from build123d import *

# Parameters (mm, degrees)
F0_R     = 30
F1_DEPTH = 10
F2_R     = 20
F3_DEPTH = 30
F4_R     = 30
F5_DEPTH = 10
F6_R     = 15
F7_DEPTH = 50


with BuildPart() as f1:
    # F0 (on Right) → F1 (new body)
    with BuildSketch(Plane.YZ):
        Circle(F0_R)
    extrude(amount=F1_DEPTH)

    # F2 (on face) → F3 (join)
    with BuildSketch(Plane.YZ.offset(10)):
        Circle(F2_R)
    extrude(amount=F3_DEPTH)

    # F4 (on face) → F5 (join)
    with BuildSketch(Plane.YZ.offset(40)):
        Circle(F4_R)
    extrude(amount=F5_DEPTH)

    # F6 (on face) → F7 (cut, through all)
    with BuildSketch(Plane.YZ.offset(50)):
        Circle(F6_R)
    extrude(amount=-F7_DEPTH, mode=Mode.SUBTRACT)


solid = f1.part
Build history of the part. All positions in model axes, mm. A direction names the side the tool comes from. Round coordinates to 2 decimals unless told otherwise and drop trailing zeros. Loops run counter-clockwise (first coordinate to the right, second up) from the corner with the lowest first, then second, coordinate; pieces in that order, holes last. Notation, with made-up numbers: (-28.5, -10) -> (-9.5, -10) arc R22 ccw to (-9.5, 11) -> close; hole circle Ø3 at (-16.75, 43.25). An arc over 180 degrees is marked (long way). One line per item, written item: value. Start each with the question number.
Q1. Drop flat-ended pins along their axis: pin 1 Ø8 at (x, z) = (33.5, -9.5) entering from -Y; pin 2 Ø1.5 at (x, y) = (19, 18) entering from -Z; pin 3 Ø4 at (x, z) = (24, -1.5) entering from +Y. Give the stop position or say it passes through.
Q2. Cut at C-C on x = 26.5. List the corners of the cut face in (y, z), plus the area to 3 significant figures.
Q3. Two-plate mould, pull along X, no slides. Class faces 3 (the face through (24.79, -4.336, -19.524)), 4 (the face through (44.93, -29.97, 1.32)), 5 (the face through (50, 6, 14)): released by +X, released by -X, zero draft, split by the parting line, or undercut.
Q4. Cut at A-A on y = 0. List the corners of the cut face in (x, z).
Q5. Cut at D-D on y = 21. List the corners of the cut face in (x, z).
Q6. 3-axis set-ups, long thin cutter, end or side, ignore diameter. For faces 1 (the face through (10, 6, -20)), 2 (the face through (25.35, -14.985, 0.66)): which of +Z, -Z, +X, -X, +Y, -Y reach the whole face in a straight line?
Q7. Probe line 1 along X through (y, z) = (-2.5, 20); line 2 along Z through (x, y) = (23, 0); line 3 along Y through (x, z) = (38, -13). List the from-to ranges inside material, lowest first.
Computed:
1. pin 1: y = -19.23
1. pin 2: z = -10.12
1. pin 3: y = 20
2. outline: circle Ø40 at (0, 0); hole circle Ø30 at (0, 0)
2. area: 550 mm²
3. face 3: undercut
3. face 4: zero draft
3. face 5: released by +X
4. outline: (0, -30) -> (10, -30) -> (10, -20) -> (40, -20) -> (40, -30) -> (50, -30) -> (50, -15) -> (0, -15) -> close; (0, 15) -> (50, 15) -> (50, 30) -> (40, 30) -> (40, 20) -> (10, 20) -> (10, 30) -> (0, 30) -> close
5. outline: (0, -21.42) -> (10, -21.42) -> (10, 21.42) -> (0, 21.42) -> close; (40, -21.42) -> (50, -21.42) -> (50, 21.42) -> (40, 21.42) -> close
6. face 1: none
6. face 2: +X, -X
7. line 1: 0 to 10, 40 to 50
7. line 2: -20 to -15, 15 to 20
7. line 3: -15.2 to -7.48, 7.48 to 15.2
